Check sheet for the modelled part. Datum: model origin and axes. Units: mm. Give positions to 0.01 mm unless a question says otherwise; leave off trailing zeros. Write each loop counter-clockwise with the first axis right and the second up, starting at its lowest first coordinate (ties: lowest second). Pieces come first, ordered by that corner, then holes. Notation, with made-up numbers: M -9.75,57 L 49.25,57 A31 ccw 49.25,90 Z; hole C 49,33 d4. An arc over 180 degrees is marked long. Use CSV: the item, a comma, the result in double quotes. Start each with the question number.
1. Cross-section at C-C, the plane z = 5. Enter the section's corners in (x, y), and give its area (3 significant figures).
2. Depth check by flat-ended pin: P1, Ø1, axis at y = 59.5, z = 5, coming from the -X side; P2, Ø1.5, axis at y = 7, z = 3.5, coming from the -X side; P3, Ø1.5, axis at x = -61, z = 1, coming from the +Y side. Enter the tip coordinate at first touch or a pass-through.
3. Scan lines: line 1 (Y direction, x = -92, z = 3); line 2 (X direction, y = -125, z = 4.25); line 3 (X direction, y = -62, z = 1). Record each from-to range of solid material in increasing order.
Autodesk Inventor part; units mm, degrees
ref_plane "YZ Plane" through (0, 0, 0) normal (1, 0, 0) x (0, 1, 0)
ref_plane "XZ Plane" through (0, 0, 0) normal (0, 1, 0) x (-1, 0, 0)
ref_plane "XY Plane" through (0, 0, 0) normal (0, 0, 1) x (1, 0, 0)
sketch "Sketch1" plane through (0, 0, 0) normal (0, 0, 1) x (1, 0, 0)
  line L0 (-180, 180) -> (180, 180)
  line L1 (180, 180) -> (180, -180)
  line L2 (180, -180) -> (-180, -180)
  line L3 (-180, -180) -> (-180, 180)
  point P0 (0, 0)
  dimension "d0" = 360
  dimension "d1" = 360
  dimension "d2" = 180
  dimension "d3" = 180
extrude "Extrusion1" add sketch "Sketch1" along normal blind 8
chamfer "Chamfer1" distance 8 angle 45 4 edges at (-180, 0, 8) (0, -180, 8) (180, 0, 8) (0, 180, 8)
equation "\"d0\" = edge_length"
equation "\"d1\" = edge_length"
equation "\"d4\" = wall_width"
equation "\"d6\" = wall_width"
properties part number "Element"
Worked answers:
1,outline,"M -175,-175 L 175,-175 L 175,175 L -175,175 Z"
1,area,"123,000 mm^2"
2,P1,"stops at x = -175.5"
2,P2,"stops at x = -177.25"
2,P3,"stops at y = 179.75"
3,line 1,"y = -177 to 177"
3,line 2,"x = -175.75 to 175.75"
3,line 3,"x = -179 to 179"
